from build123d import *

# Parameters (mm, degrees)
SKETCH_1_R      = 2.5
SKETCH_1_R_2    = 3
EXTRUDE_1_DEPTH = 1000


with BuildPart() as part:
    # Эскиз1 → Бобышка-Вытянуть1 (new body)
    with BuildSketch(Plane.XY):
        with BuildLine():
            Line((-15, 5.45), (-15, 14))
            ThreePointArc((-15, 14), (-14.707106781, 14.707106781), (-14, 15))
            Line((-14, 15), (-5.45, 15))
            Line((-5.45, 15), (-3.25, 15))
            Line((-3.25, 15), (-3.25, 13.2))
            Line((-3.25, 13.2), (-5.45, 13.2))
            Line((-5.45, 13.2), (-5.45, 7))
            ThreePointArc((-5.45, 7), (0, 5.022844472), (5.45, 7))
            Line((5.45, 7), (5.45, 13.2))
            Line((5.45, 13.2), (3.25, 13.2))
            Line((3.25, 13.2), (3.25, 15))
            Line((3.25, 15), (5.45, 15))
            Line((5.45, 15), (14, 15))
            ThreePointArc((14, 15), (14.707106781, 14.707106781), (15, 14))
            Line((15, 14), (15, 5.45))
            Line((15, 5.45), (15, 3.25))
            Line((15, 3.25), (13.2, 3.25))
            Line((13.2, 3.25), (13.2, 5.45))
            Line((13.2, 5.45), (7, 5.45))
            ThreePointArc((7, 5.45), (5.022844472, 0), (7, -5.45))
            Line((7, -5.45), (13.2, -5.45))
            Line((13.2, -5.45), (13.2, -3.25))
            Line((13.2, -3.25), (15, -3.25))
            Line((15, -3.25), (15, -5.45))
            Line((15, -5.45), (15, -24.55))
            Line((15, -24.55), (15, -26.75))
            Line((15, -26.75), (13.2, -26.75))
            Line((13.2, -26.75), (13.2, -24.55))
            Line((13.2, -24.55), (7, -24.55))
            ThreePointArc((7, -24.55), (5.022844472, -30), (7, -35.45))
            Line((7, -35.45), (13.2, -35.45))
            Line((13.2, -35.45), (13.2, -33.25))
            Line((13.2, -33.25), (15, -33.25))
            Line((15, -33.25), (15, -35.45))
            Line((15, -35.45), (15, -44))
            ThreePointArc((15, -44), (14.707106781, -44.707106781), (14, -45))
            Line((14, -45), (5.45, -45))
            Line((5.45, -45), (3.25, -45))
            Line((3.25, -45), (3.25, -43.2))
            Line((3.25, -43.2), (5.45, -43.2))
            Line((5.45, -43.2), (5.45, -37))
            ThreePointArc((5.45, -37), (0, -35.022844472), (-5.45, -37))
            Line((-5.45, -37), (-5.45, -43.2))
            Line((-5.45, -43.2), (-3.25, -43.2))
            Line((-3.25, -43.2), (-3.25, -45))
            Line((-3.25, -45), (-5.45, -45))
            Line((-5.45, -45), (-14, -45))
            ThreePointArc((-14, -45), (-14.707106781, -44.707106781), (-15, -44))
            Line((-15, -44), (-15, -35.45))
            Line((-15, -35.45), (-15, -33.25))
            Line((-15, -33.25), (-13.2, -33.25))
            Line((-13.2, -33.25), (-13.2, -35.45))
            Line((-13.2, -35.45), (-7, -35.45))
            ThreePointArc((-7, -35.45), (-5.022844472, -30), (-7, -24.55))
            Line((-7, -24.55), (-13.2, -24.55))
            Line((-13.2, -24.55), (-13.2, -26.75))
            Line((-13.2, -26.75), (-15, -26.75))
            Line((-15, -26.75), (-15, -24.55))
            Line((-15, -24.55), (-15, -5.45))
            Line((-15, -5.45), (-15, -3.25))
            Line((-15, -3.25), (-13.2, -3.25))
            Line((-13.2, -3.25), (-13.2, -5.45))
            Line((-13.2, -5.45), (-7, -5.45))
            ThreePointArc((-7, -5.45), (-5.022844472, 0), (-7, 5.45))
            Line((-7, 5.45), (-13.2, 5.45))
            Line((-13.2, 5.45), (-13.2, 3.25))
            Line((-13.2, 3.25), (-15, 3.25))
            Line((-15, 3.25), (-15, 5.45))
        make_face()
        Circle(SKETCH_1_R, mode=Mode.SUBTRACT)
        with Locations((0, -30)):
            Circle(SKETCH_1_R, mode=Mode.SUBTRACT)
        with Locations((-9.5, 10.25)):
            Circle(SKETCH_1_R_2, mode=Mode.SUBTRACT)
        with Locations((9.5, 10.25)):
            Circle(SKETCH_1_R_2, mode=Mode.SUBTRACT)
        with Locations((-9.5, -40.25)):
            Circle(SKETCH_1_R_2, mode=Mode.SUBTRACT)
        with Locations((9.5, -40.25)):
            Circle(SKETCH_1_R_2, mode=Mode.SUBTRACT)
        with BuildLine():
            Line((-13, -22.5), (-13, -7.5))
            Line((-13, -7.5), (-5.830951895, -7.5))
            ThreePointArc((-5.830951895, -7.5), (0, -5.5), (5.830951895, -7.5))
            Line((5.830951895, -7.5), (13, -7.5))
            Line((13, -7.5), (13, -22.5))
            Line((13, -22.5), (5.830951895, -22.5))
            ThreePointArc((5.830951895, -22.5), (0, -24.5), (-5.830951895, -22.5))
            Line((-5.830951895, -22.5), (-13, -22.5))
        make_face(mode=Mode.SUBTRACT)
    extrude(amount=EXTRUDE_1_DEPTH)


solid = part.part
CAD build for the part. Positions are in the model's coordinates, mm. Give positions to 0.01 mm unless a question says otherwise; leave off trailing zeros. Put each result on its own line as item: value. Start each with the question number.
(1) Band-saw the part on A-A, the plane z = 681.5. Give the number of separate pieces and of enclosed holes in the cut face, and give its area (3 significant figures).
(2) Flat gauge pin, fed straight in: pin 1 Ø2 at (x, z) = (-2, 727.5) entering from -Y. Where does the tip first touch, or does it go through?
(3) Probe L1, parallel to Y at x = -9.5, z = 640; L2, parallel to X at y = -40, z = 628; L3, parallel to Y at x = 0, z = 397. List the from-to ranges inside material, lowest first.
Response values:
1. separate pieces: 1
1. enclosed holes: 7
1. area: 661 mm2
2. pin 1: stops at y = -35.57
3. L1: y = -45 to -43.25, -37.25 to -35.45, -24.55 to -22.5, -7.5 to -5.45, 5.45 to 7.25, 13.25 to 15
3. L2: x = -15 to -12.49, -6.51 to -5.45, 5.45 to 6.51, 12.49 to 15
3. L3: y = -35.02 to -32.5, -27.5 to -24.5, -5.5 to -2.5, 2.5 to 5.02
